```python
from build123d import *

# Parameters (mm, degrees)
SKETCH275_R             = 3.75
PAD158_DEPTH            = 10
SKETCH276_R             = 5.75
PAD159_DEPTH            = 2.5
SKETCH277_R             = 2.95
POCKET130_DEPTH         = 1.1
SKETCH278_R             = 2.45
POCKET131_DEPTH         = 3.6
POCKET132_DEPTH         = 1
CHAMFER_SIZE            = 0.5
SKETCH280_W             = 4
SKETCH280_H             = 4
POCKET133_DEPTH         = 6.25
BODY023_PLACEMENT_ANGLE = 180


with BuildPart() as part:
    # Sketch275 → Pad158 (new body)
    with BuildSketch(Plane.XY):
        Circle(SKETCH275_R)
    extrude(amount=PAD158_DEPTH)

    # Sketch276 (on Face3 of Pad158) → Pad159 (join)
    with BuildSketch(Plane.XY.offset(10)):
        Circle(SKETCH276_R)
    extrude(amount=PAD159_DEPTH)

    # Sketch277 (on Face5 of Pad159) → Pocket130 (cut)
    with BuildSketch(Plane.XY.offset(12.5)):
        Circle(SKETCH277_R)
    extrude(amount=-POCKET130_DEPTH, mode=Mode.SUBTRACT)

    # Sketch278 (on Face7 of Pocket130) → Pocket131 (cut)
    with BuildSketch(Plane.XY.offset(11.4)):
        Circle(SKETCH278_R)
    extrude(amount=-POCKET131_DEPTH, mode=Mode.SUBTRACT)

    # Sketch279 (on Face5 of Pocket131) → Pocket132 (cut)
    with BuildSketch(Plane.XY.offset(12.5)):
        Polygon((-0.5, 6.25), (-0.5, 1.25), (-4.035534, 4.785534), (-4.742641, 4.078427), (-1.164214, 0.5), (-6.164214, 0.5), (-6.164214, -0.5), (-1.164214, -0.5), (-4.699747, -4.035534), (-3.992641, -4.742641), (-0.5, -1.25), (-0.5, -6.25), (0.5, -6.25), (0.5, -1.25), (3.992641, -4.742641), (4.699747, -4.035534), (1.164214, -0.5), (6.164214, -0.5), (6.164214, 0.5), (1.164214, 0.5), (4.742641, 4.078427), (4.035534, 4.785534), (0.5, 1.25), (0.5, 6.25), align=None)
    extrude(amount=-POCKET132_DEPTH, mode=Mode.SUBTRACT)

    # Chamfer
    chamfer_edges = [part.edges().sort_by_distance(p)[0] for p in [
        (0.5, 4.317769, 12.5),
        (-0.5, 4.317769, 12.5),
        (-2.675257, 3.425257, 12.5),
        (-3.387925, 2.723711, 12.5),
        (-4.317769, 0.5, 12.5),
        (-4.317769, -0.5, 12.5),
        (-3.387925, -2.723711, 12.5),
        (-2.675257, -3.425257, 12.5),
        (-0.5, -4.317769, 12.5),
        (0.5, -4.317769, 12.5),
        (2.675257, -3.425257, 12.5),
        (3.387925, -2.723711, 12.5),
        (4.317769, -0.5, 12.5),
        (4.317769, 0.5, 12.5),
        (3.387925, 2.723711, 12.5),
        (2.675257, 3.425257, 12.5),
    ]]
    chamfer(chamfer_edges, length=CHAMFER_SIZE)

    # Sketch280 (on Face54 of Chamfer) → Pocket133 (cut)
    with BuildSketch(Plane(origin=(0, 0, 0), x_dir=(1, 0, 0), z_dir=(0, 0, -1))):
        Rectangle(SKETCH280_W, SKETCH280_H)
    extrude(amount=-POCKET133_DEPTH, mode=Mode.SUBTRACT)


with BuildPart() as part_1:
    # Body023 placement: moved
    add(part.part.moved(Location((38.2, -32, -11))).rotate(Axis((38.2, -32, -11), (0, 0, 1)), BODY023_PLACEMENT_ANGLE))


solid = part_1.part
```
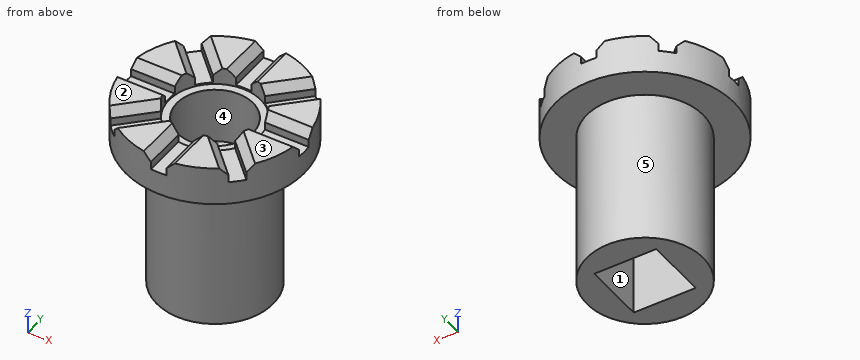
Design review of the part built by this model. Coordinates are the model's own, in mm. Face numbers are marked on the shaded views. A direction names the side the tool comes from. Round coordinates to 2 decimals unless told otherwise and drop trailing zeros. Write each loop counter-clockwise with the first axis right and the second up, starting at its lowest first coordinate (ties: lowest second). Pieces come first, ordered by that corner, then holes.
Item 1: We need section D-D on z = -7.25. Write out the cut boundary in (x, y).
Item 2: We need section C-C on z = -1.75. Write out the cut boundary in (x, y), and give its area (3 significant figures).
Item 3: Clearance check with flat-ended pins moving along their axes: pin 1 Ø2 at (y, z) = (-32, -6.5) entering from +X; pin 2 Ø1.2 at (x, z) = (39, -7) entering from +Y; pin 3 Ø1.5 at (y, z) = (-34, -2) entering from +X. State where each tip first meets the part, or that it passes through.
Item 4: For probe 1 along Y at (x, z) = (38.2, -1.2); probe 2 along Z at (x, y) = (33.5, -31.75); probe 3 along Z at (x, y) = (39, -33.25), list the stretches that pass through material, from the lowest coordinate up.
Item 5: We need section B-B on x = 38.2. Write out the cut boundary in (y, z).
Item 6: For the marked faces 1 and 2, list the 3-axis set-ups (+Z, -Z, +X, -X, +Y, -Y) from which the entire face can be reached by the end or side of a thin tool; tool diameter is ignored.
Item 7: The part is to be moulded in two halves that separate along X. For the marked faces 3, 4 and 5, say which applies: +X half, -X half, draft (parallel to the pull), parting line (faces both ways), or undercut.
Item 8: We need section A-A on y = -32. Write out the cut boundary in (x, z).
Returned:
1. outline: circle Ø7.5 at (38.2, -32); hole (36.2, -34) - (40.2, -34) - (40.2, -30) - (36.2, -30) - close
2. outline: circle Ø7.5 at (38.2, -32); hole circle Ø4.9 at (38.2, -32)
2. area: 25.3 mm2
3. pin 1: stops at x = 41.95
3. pin 2: stops at y = -28.26
3. pin 3: stops at x = 41.74
4. probe 1: y = -35.75 to -34.45, -29.55 to -28.25
4. probe 2: z = -1 to 0.5
4. probe 3: z = -4.75 to -3.2
5. outline: (-37.75, -1) - (-35.75, -1) - (-35.75, -11) - (-34, -11) - (-34, -4.75) - (-30, -4.75) - (-30, -11) - (-28.25, -11) - (-28.25, -1) - (-26.25, -1) - (-26.25, 0.5) - (-29.05, 0.5) - (-29.05, 0.4) - (-29.55, 0.4) - (-29.55, -3.2) - (-34.45, -3.2) - (-34.45, 0.4) - (-34.95, 0.4) - (-34.95, 0.5) - (-37.75, 0.5) - close
6. face 1: -Z
6. face 2: +Z, +X, -X, +Y, -Y
7. face 3: draft
7. face 4: undercut
7. face 5: parting line
8. outline: (32.45, -1) - (34.45, -1) - (34.45, -11) - (36.2, -11) - (36.2, -4.75) - (40.2, -4.75) - (40.2, -11) - (41.95, -11) - (41.95, -1) - (43.95, -1) - (43.95, 0.5) - (41.15, 0.5) - (41.15, 0.4) - (40.65, 0.4) - (40.65, -3.2) - (35.75, -3.2) - (35.75, 0.4) - (35.25, 0.4) - (35.25, 0.5) - (32.45, 0.5) - close
